```python
from build123d import *

# Parameters (mm, degrees)
SKETCH2_R           = 5.08
BOSS_EXTRUDE1_DEPTH = 35.56
SKETCH4_R           = 7.62
BOSS_EXTRUDE2_DEPTH = 1.778
SKETCH5_R           = 3.175
CUT_EXTRUDE2_DEPTH  = 39.862
CUT_EXTRUDE3_DEPTH  = 35.56


with BuildPart() as part:
    # Sketch2 → Boss-Extrude1 (new body)
    with BuildSketch(Plane(origin=(0, 0, 0), x_dir=(1, 0, 0), z_dir=(0, 1, 0))):
        with Locations(Location((0, 0, 0), (0, 0, 270))):
            Circle(SKETCH2_R)
    extrude(amount=BOSS_EXTRUDE1_DEPTH)

    # Sketch4 → Boss-Extrude2 (add)
    with BuildSketch(Plane(origin=(0, 35.56, 0), x_dir=(1, 0, 0), z_dir=(0, 1, 0))):
        with Locations(Location((0, 0, 0), (0, 0, 270))):
            Circle(SKETCH4_R)
    extrude(amount=BOSS_EXTRUDE2_DEPTH)

    # Sketch5 → Cut-Extrude2 (cut, through all)
    with BuildSketch(Plane(origin=(0, 37.338, 0), x_dir=(1, 0, 0), z_dir=(0, 1, 0))):
        with Locations(Location((0, 0, 0), (0, 0, 270))):
            Circle(SKETCH5_R)
    extrude(amount=-CUT_EXTRUDE2_DEPTH, mode=Mode.SUBTRACT)

    # Sketch6 → Cut-Extrude3 (cut)
    with BuildSketch(Plane.XZ):
        with BuildLine():
            Line((-3.77856884, 3.395411245), (-3.542408287, 3.183198042))
            ThreePointArc((-3.542408287, 3.183198042), (-4.399976274, 1.822529847), (-4.755721843, 0.254))
            Line((-4.755721843, 0.254), (-5.072769966, 0.270933333))
            ThreePointArc((-5.072769966, 0.270933333), (-4.693308025, 1.944031836), (-3.77856884, 3.395411245))
        make_face()
        with BuildLine():
            Line((-0.270933333, 5.072769966), (-0.254, 4.755721843))
            ThreePointArc((-0.254, 4.755721843), (-1.822529847, 4.399976274), (-3.183198042, 3.542408287))
            Line((-3.183198042, 3.542408287), (-3.395411245, 3.77856884))
            ThreePointArc((-3.395411245, 3.77856884), (-1.944031836, 4.693308025), (-0.270933333, 5.072769966))
        make_face()
        with BuildLine():
            Line((0.270933333, 5.072769966), (0.254, 4.755721843))
            ThreePointArc((0.254, 4.755721843), (1.822529847, 4.399976274), (3.183198042, 3.542408287))
            Line((3.183198042, 3.542408287), (3.395411245, 3.77856884))
            ThreePointArc((3.395411245, 3.77856884), (1.944031836, 4.693308025), (0.270933333, 5.072769966))
        make_face()
        with BuildLine():
            Line((3.77856884, 3.395411245), (3.542408287, 3.183198042))
            ThreePointArc((3.542408287, 3.183198042), (4.399976274, 1.822529847), (4.755721843, 0.254))
            Line((4.755721843, 0.254), (5.072769966, 0.270933333))
            ThreePointArc((5.072769966, 0.270933333), (4.693308025, 1.944031836), (3.77856884, 3.395411245))
        make_face()
        with BuildLine():
            Line((5.072769966, -0.270933333), (4.755721843, -0.254))
            ThreePointArc((4.755721843, -0.254), (4.399976274, -1.822529847), (3.542408287, -3.183198042))
            Line((3.542408287, -3.183198042), (3.77856884, -3.395411245))
            ThreePointArc((3.77856884, -3.395411245), (4.693308025, -1.944031836), (5.072769966, -0.270933333))
        make_face()
        with BuildLine():
            Line((3.183198042, -3.542408287), (3.395411245, -3.77856884))
            ThreePointArc((3.395411245, -3.77856884), (1.944031836, -4.693308025), (0.270933333, -5.072769966))
            Line((0.270933333, -5.072769966), (0.254, -4.755721843))
            ThreePointArc((0.254, -4.755721843), (1.822529847, -4.399976274), (3.183198042, -3.542408287))
        make_face()
        with BuildLine():
            Line((-4.755721843, -0.254), (-5.072769966, -0.270933333))
            ThreePointArc((-5.072769966, -0.270933333), (-4.693308025, -1.944031836), (-3.77856884, -3.395411245))
            Line((-3.77856884, -3.395411245), (-3.542408287, -3.183198042))
            ThreePointArc((-3.542408287, -3.183198042), (-4.399976274, -1.822529847), (-4.755721843, -0.254))
        make_face()
        with BuildLine():
            Line((-3.183198042, -3.542408287), (-3.395411245, -3.77856884))
            ThreePointArc((-3.395411245, -3.77856884), (-1.944031836, -4.693308025), (-0.270933333, -5.072769966))
            Line((-0.270933333, -5.072769966), (-0.254, -4.755721843))
            ThreePointArc((-0.254, -4.755721843), (-1.822529847, -4.399976274), (-3.183198042, -3.542408287))
        make_face()
    extrude(amount=-CUT_EXTRUDE3_DEPTH, mode=Mode.SUBTRACT)


solid = part.part
```
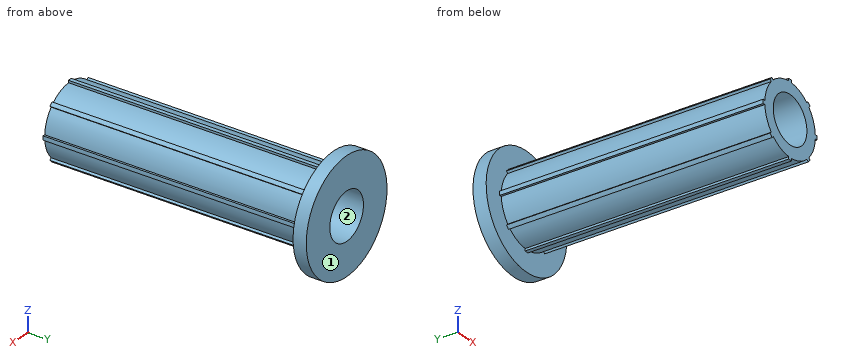
Geometry: final body of the model. Coordinates: model frame, mm. Face numbers are marked on the shaded views. Round coordinates to 2 decimals unless told otherwise and drop trailing zeros. Write each loop counter-clockwise with the first axis right and the second up, starting at its lowest first coordinate (ties: lowest second). Pieces come first, ordered by that corner, then holes. Notation, with made-up numbers: (71, -16.5) -> (106, -16.5) arc R25 ccw to (106, 18.5) -> close; hole circle Ø1 at (12, 3). An arc over 180 degrees is marked (long way). Return JSON: item names as keys, results as strings.
Q1. Mould query, pull axis Z, two halves, no side actions, for the marked faces 1 and 2. Classes: +Z half, -Z half, draft (parallel to the pull), parting line (faces both ways), or undercut.
From the geometry:
{"face 1": "draft", "face 2": "undercut"}
Q2. Section C-C on z = -2. Return the cut outline in (x, y), and give its area (3 significant figures).
From the geometry:
{"outline": "(-7.35, 35.56) -> (-4.32, 35.56) -> (-4.32, 0) -> (-2.47, 0) -> (-2.47, 37.34) -> (-7.35, 37.34) -> close; (2.47, 0) -> (4.32, 0) -> (4.32, 35.56) -> (7.35, 35.56) -> (7.35, 37.34) -> (2.47, 37.34) -> close", "area": "149 mm2"}
Q3. First-contact query: pin 1 Ø5 at (y, z) = (10.5, -0.5) entering from -X; pin 2 Ø3 at (y, z) = (6.5, 3.5) entering from -X; pin 3 Ø8 at (x, y) = (5.5, 14) entering from -Z. Flat tips, straight axial feed; report the tip coordinate or a pass-through.
From the geometry:
{"pin 1": "x = -5.08", "pin 2": "x = -4.32", "pin 3": "z = -4.52"}
Q4. Section D-D on z = -6. Return the cut outline in (x, y), and give its area (3 significant figures).
From the geometry:
{"outline": "(-4.7, 35.56) -> (4.7, 35.56) -> (4.7, 37.34) -> (-4.7, 37.34) -> close", "area": "16.7 mm2"}
Q5. Section B-B on x = -1.5. Return the cut outline in (y, z), and give its area (3 significant figures).
From the geometry:
{"outline": "(0, -4.52) -> (35.56, -4.52) -> (35.56, -7.47) -> (37.34, -7.47) -> (37.34, -2.8) -> (0, -2.8) -> close; (0, 2.8) -> (37.34, 2.8) -> (37.34, 7.47) -> (35.56, 7.47) -> (35.56, 4.52) -> (0, 4.52) -> close", "area": "139 mm2"}
Q6. Ray query, line 1 (Y direction, x = 2.25, z = 4.5); line 2 (X direction, y = 31.5, z = 2); line 3 (X direction, y = 18.5, z = -2.5). Return the intervals inside material, ascending.
From the geometry:
{"line 1": "35.56 to 37.34", "line 2": "-4.32 to -2.47, 2.47 to 4.32", "line 3": "-4.05 to -1.96, 1.96 to 4.05"}
